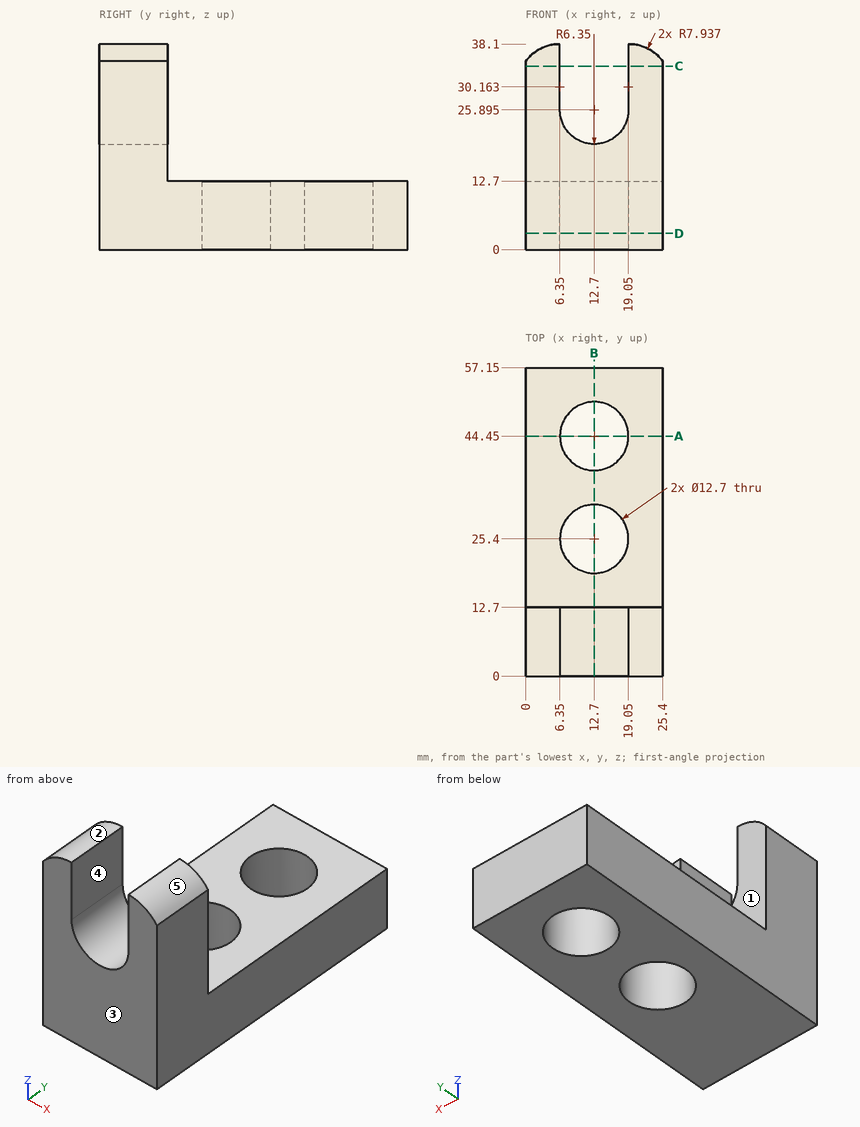
The drawing under review shows one solid part. Ordinate dimensions are in mm from its lowest x, y, z. A direction names the side the tool comes from. Coordinates: 2 decimals unless noted, no trailing zeros. Write each loop counter-clockwise with the first axis right and the second up, starting at its lowest first coordinate (ties: lowest second). Pieces come first, ordered by that corner, then holes. Notation, with made-up numbers: (55, 85) - (80, 85) arc R18 cw to (80, 94) - close; hole circle Ø4 at (47, 25). An arc over 180 degrees is marked (long way). Answer in a Markdown table with one row per item. Add a question column.
Q1. Tool access review of the marked faces 1 and 2: name each direction out of +Z, -Z, +X, -X, +Y, -Y from which nothing blocks a thin tool from reaching the whole face with its end or side.
Q2. We need section A-A, the plane y = 44.45. State the section outline as (x, z) points.
Q3. For P1, Ø12.5, axis at x = 17, z = 23.5, coming from the +Y side; P2, Ø10, axis at x = 19, y = 21, coming from the +Z side, all flat-tipped, find the tip position at first contact; note any pin that passes through.
Q4. Draft analysis for pull direction X (two halves, no side actions). For the marked faces 3, 4 and 5, state which applies: +X half, -X half, draft (parallel to the pull), parting line (faces both ways), or undercut.
Q5. For probe 1 along Y at (x, z) = (12.7, 6); probe 2 along Y at (x, z) = (17.75, 6.5); probe 3 along Z at (x, y) = (16.5, 19), list the stretches that pass through material, from the lowest coordinate up.
Q6. We need section D-D, the plane z = 3. State the section outline as (x, y) points, and give its area (3 significant figures).
Q7. We need section B-B, the plane x = 12.7. Count the separate pieces of the cut face and the enclosed holes in it, and give its area (3 significant figures).
Answer list:
| question | item | result |
|---|---|---|
| 1 | face 1 | +Z, +X, -X, +Y |
| 1 | face 2 | +Z, -X, +Y, -Y |
| 2 | outline | (0, 0) - (6.35, 0) - (6.35, 12.7) - (0, 12.7) - close; (19.05, 0) - (25.4, 0) - (25.4, 12.7) - (19.05, 12.7) - close |
| 3 | P1 | stops at y = 12.7 |
| 3 | P2 | stops at z = 12.7 |
| 4 | face 3 | draft |
| 4 | face 4 | undercut |
| 4 | face 5 | +X half |
| 5 | probe 1 | y = 0 to 19.05, 31.75 to 38.1, 50.8 to 57.15 |
| 5 | probe 2 | y = 0 to 21.55, 29.25 to 40.6, 48.3 to 57.15 |
| 5 | probe 3 | z = 0 to 12.7 |
| 6 | outline | (0, 0) - (25.4, 0) - (25.4, 57.15) - (0, 57.15) - close; hole circle Ø12.7 at (12.7, 25.4); hole circle Ø12.7 at (12.7, 44.45) |
| 6 | area | 1,200 mm2 |
| 7 | separate pieces | 3 |
| 7 | enclosed holes | 0 |
| 7 | area | 490 mm2 |
